Model file for the job. Use its own axes, mm. A direction names the side the tool comes from. Give positions to 0.01 mm unless a question says otherwise; leave off trailing zeros. Loops run counter-clockwise (first coordinate to the right, second up) from the corner with the lowest first, then second, coordinate; pieces in that order, holes last. Notation, with made-up numbers: (-3.75, -39.5) -> (36.25, -39.5) arc R38 cw to (36.25, -0.5) -> close; hole circle Ø7 at (80, 56). An arc over 180 degrees is marked (long way). Use CSV: the item, a comma, the result in double quotes. Start each with the question number.
(1) 3-axis set-ups, long thin cutter, end or side, ignore diameter. For faces 1 (the flat face through (-1, -73, 2)), 2 (the flat face through (59, 0, 0)): which of +Z, -Z, +X, -X, +Y, -Y reach the whole face in a straight line?
(2) Cut at A-A on y = -55. Write the cut outline in (x, z), then the cut area to 3 significant figures.
(3) Cut at C-C on z = 1.7. Write the cut outline in (x, y), then the cut area to 3 significant figures.
(4) Flat gauge pin, fed straight in: pin 1 (6.5 mm diameter, centred on x = 55, y = -74, fed in from +Z) (1 decimal). Where does the tip first touch, or does it go through?
(5) Pull direction Y, two halves, no side cores. Call faces 3 (the cylindrical face through (-61, 79, 2)), 4 (the cylindrical face through (51.72, -68.49, 2.46)), 5 (the flat face through (59, 0, 5)): pulls with the +Y half, pulls with the -Y half, needs draft (parallel to the pull), parting line crosses it, or undercut.
(6) Drill centre lines: probe 1 along Y at (x, z) = (0, 1.8); probe 2 along Y at (x, z) = (13, 0.4); probe 3 along X at (y, z) = (29.5, 2.25). Where is each one in solid material? Low to high.
(7) Cut at B-B on x = -4. Write the cut outline in (y, z).
Autodesk Inventor part; units mm, degrees
ref_plane "YZ Plane" through (0, 0, 0) normal (1, 0, 0) x (0, 1, 0)
ref_plane "XZ Plane" through (0, 0, 0) normal (0, 1, 0) x (-1, 0, 0)
ref_plane "XY Plane" through (0, 0, 0) normal (0, 0, 1) x (1, 0, 0)
sketch "Sketch1" plane through (0, 0, 0) normal (0, 0, 1) x (1, 0, 0)
  line L0 (-57, -81) -> (57, -81)
  line L1 (62, -76) -> (62, -22)
  line L2 (57, 81) -> (-57, 81)
  line L3 (-62, 76) -> (-62, 9)
  line L4 (-41, -73) -> (41, -73)
  line L5 (56, -58) -> (56, -22)
  line L6 (41, 73) -> (-41, 73)
  line L7 (-56, 58) -> (-56, 9)
  arc A0 (-56, -58) -> (-41, -73) centre (-41, -58) ccw
  arc A1 (-41, 73) -> (-56, 58) centre (-41, 58) ccw
  arc A2 (56, 58) -> (41, 73) centre (41, 58) ccw
  arc A3 (41, -73) -> (56, -58) centre (41, -58) ccw
  line L8 (56, -22) -> (62, -22) construction
  line L9 (56, -10) -> (62, -10) construction
  line L10 (-56, 9) -> (-62, 9)
  line L11 (-62, -22) -> (-56, -22) construction
  line L12 (-62, -22) -> (-62, -76)
  line L13 (-62, 9) -> (-62, -9) construction
  line L14 (-56, -22) -> (-56, -58)
  line L15 (-56, 9) -> (-56, -9) construction
  line L16 (56, -22) -> (56, -10)
  line L17 (56, -10) -> (56, 58)
  line L18 (62, -22) -> (62, -10)
  line L19 (62, -10) -> (62, 76)
  arc A4 (-62, -76) -> (-57, -81) centre (-57, -76) ccw
  arc A5 (-57, 81) -> (-62, 76) centre (-57, 76) ccw
  arc A6 (62, 76) -> (57, 81) centre (57, 76) ccw
  arc A7 (57, -81) -> (62, -76) centre (57, -76) ccw
  circle A8 centre (-55, -74) radius 5.25
  line L20 (-92.4325, 0) -> (79.0499, 0) construction
  line L21 (0, -100.3717) -> (0, 120.689) construction
  circle A9 centre (-55, 74) radius 5.25
  circle A10 centre (55, -74) radius 5.25
  circle A11 centre (55, 74) radius 5.25
  line L22 (-56, -9) -> (-62, -9)
  line L23 (-62, -9) -> (-62, -22)
  line L24 (-56, -9) -> (-56, -22)
  circle A12 centre (0, -77) radius 2.1
  point P0 (0, 0)
  point P1 (-62, -81)
  point P2 (62, 81)
  point P3 (-62, 81)
  dimension "d0" = 162
  dimension "d1" = 124
  dimension "d2" = 62
  dimension "d3" = 81
  dimension "d4" = 6
  dimension "d5" = 8
  dimension "d6" = 6
  dimension "d7" = 8
  dimension "d8" = 15
  dimension "d9" = 12
  dimension "d10" = 59
  dimension "d11" = 59
  dimension "d12" = 72
  dimension "d13" = 5
  dimension "d14" = 7
  dimension "d15" = 7
  dimension "d16" = 10.5
  dimension "d19" = 72
  dimension "d21" = 4
  dimension "d22" = 4.2
extrude "Extrusion1" add sketch "Sketch1" along normal blind 5
fillet "Fillet1" radius 2 2 edges at (-62, 9, 2.5) (-62, -9, 2.5)
properties part number "Plex_Rand_untere2" material "PET Plastic"
Check result:
1,face 1,"+Z, -Z"
1,face 2,"-Z, +X, -X, +Y, -Y"
2,outline,"(-62, 0) -> (-56, 0) -> (-56, 5) -> (-62, 5) -> close; (56, 0) -> (62, 0) -> (62, 5) -> (56, 5) -> close"
2,area,"60.0 mm²"
3,outline,"(-62, -76) arc R5 ccw to (-57, -81) -> (57, -81) arc R5 ccw to (62, -76) -> (62, 76) arc R5 ccw to (57, 81) -> (-57, 81) arc R5 ccw to (-62, 76) -> (-62, 11) arc R2 ccw to (-60, 9) -> (-56, 9) -> (-56, 58) arc R15 cw to (-41, 73) -> (41, 73) arc R15 cw to (56, 58) -> (56, -58) arc R15 cw to (41, -73) -> (-41, -73) arc R15 cw to (-56, -58) -> (-56, -9) -> (-60, -9) arc R2 ccw to (-62, -11) -> close; hole circle Ø10.5 at (-55, -74); hole circle Ø10.5 at (-55, 74); hole circle Ø4.2 at (0, -77); hole circle Ø10.5 at (55, -74); hole circle Ø10.5 at (55, 74)"
3,area,"3,440 mm²"
4,pin 1,"through"
5,face 3,"pulls with the +Y half"
5,face 4,"undercut"
5,face 5,"needs draft"
6,probe 1,"-81 to -79.1, -74.9 to -73, 73 to 81"
6,probe 2,"-81 to -73, 73 to 81"
6,probe 3,"-62 to -56, 56 to 62"
7,outline,"(-81, 0) -> (-73, 0) -> (-73, 5) -> (-81, 5) -> close; (73, 0) -> (81, 0) -> (81, 5) -> (73, 5) -> close"
